Here's how the part is built. I have some questions about the finished solid (model axes, mm). A direction names the side the tool comes from. Round coordinates to 2 decimals unless told otherwise and drop trailing zeros. Order: outer loops, then holes, each group sorted by start corner. A loop starts at its lowest first (then second) coordinate and runs counter-clockwise, first axis right, second up.
```python
from build123d import *

# Parameters (mm, degrees)
SKETCH1_R           = 14
SKETCH1_R_2         = 5
BOSS_EXTRUDE1_DEPTH = 38
SKETCH2_R           = 6.35
SKETCH2_R_2         = 3.25
BOSS_EXTRUDE2_DEPTH = 12
SKETCH3_R           = 2.5
CUT_EXTRUDE6_DEPTH  = 10


with BuildPart() as part:
    # Sketch1 → Boss-Extrude1 (new body)
    with BuildSketch(Plane(origin=(0, 0, 0), x_dir=(1, 0, 0), z_dir=(0, 1, 0))):
        with BuildLine():
            Line((40, 57), (-40, 57))
            ThreePointArc((-40, 57), (-58.987886037, 46.111263827), (-59.17994648, 24.223653075))
            Line((-59.17994648, 24.223653075), (-47.255332989, 3))
            Line((-47.255332989, 3), (-32.311027529, 3))
            ThreePointArc((-32.311027529, 3), (32.415238263, -1.501608583), (-32.45, 0))
            Line((-32.45, 0), (-47.255332989, 0))
            Line((-47.255332989, 0), (-47.255332989, -10))
            Line((-47.255332989, -10), (-41.255332989, -10))
            ThreePointArc((-41.255332989, -10), (-4.643586709, -42.195255687), (38.093342034, -18.732319468))
            Line((38.093342034, -18.732319468), (59.742132503, 25.291848568))
            ThreePointArc((59.742132503, 25.291848568), (58.675911377, 46.627997861), (40, 57))
        make_face()
        with Locations((-40, 35)):
            Circle(SKETCH1_R, mode=Mode.SUBTRACT)
        with Locations((0, 44)):
            Circle(SKETCH1_R_2, mode=Mode.SUBTRACT)
        with Locations((40, 35)):
            Circle(SKETCH1_R, mode=Mode.SUBTRACT)
    extrude(amount=BOSS_EXTRUDE1_DEPTH)


with BuildPart() as body_2:
    # Sketch2 → Boss-Extrude2 (new body)
    with BuildSketch(Plane(origin=(0, 38, 0), x_dir=(1, 0, 0), z_dir=(0, 1, 0))):
        with BuildLine():
            Line((-40, 27), (40, 27))
            ThreePointArc((40, 27), (45.282843577, 28.992374534), (47.934336402, 33.977109066))
            Line((47.934336402, 33.977109066), (50, 50))
            Line((50, 50), (50, 58))
            Line((50, 58), (-50, 58))
            Line((-50, 58), (-50, 50))
            Line((-50, 50), (-47.934336402, 33.977109066))
            ThreePointArc((-47.934336402, 33.977109066), (-45.282843577, 28.992374534), (-40, 27))
        make_face()
        with Locations((0, 44)):
            Circle(SKETCH2_R, mode=Mode.SUBTRACT)
        with Locations((-40, 35)):
            Circle(SKETCH2_R_2, mode=Mode.SUBTRACT)
        with Locations((40, 35)):
            Circle(SKETCH2_R_2, mode=Mode.SUBTRACT)
    extrude(amount=BOSS_EXTRUDE2_DEPTH)

    # Sketch3 → Cut-Extrude6 (cut)
    with BuildSketch(Plane(origin=(0, 0, -58), x_dir=(-1, 0, 0), z_dir=(0, 0, -1))):
        with Locations((0, 44)):
            Circle(SKETCH3_R)
        with Locations((40, 44)):
            Circle(SKETCH3_R)
        with Locations((-40, 44)):
            Circle(SKETCH3_R)
    extrude(amount=-CUT_EXTRUDE6_DEPTH, mode=Mode.SUBTRACT)


solid = body_2.part
```
1) We'd pull the mould along Y, two halves only. Please class faces 1 (the cylindrical face through (-38.5, 43.916, -32.117)), 2 (the flat face through (-1, 50, -36)), 3 (the flat face through (-40, 44, -48)): +Y half, -Y half, draft (parallel to the pull), parting line (faces both ways), or undercut.
2) I need wall thicknesses on line 1 (Z direction, x = 0, y = 41.25); line 2 (Y direction, x = -40, z = -54); line 3 (X direction, y = 49.75, z = -36.5). Which ranges of each line are inside material? Lowest first, please.
3) If we section it at D-D (y = 44): Write out the boundary of the cut face in (x, z).
4) I'm going to push flat-ended pins straight in: pin 1 (16.5 mm diameter, centred on x = 0, z = -44, fed in from -Y); pin 2 (1 mm diameter, centred on y = 44, z = -46, fed in from -X); pin 3 (4 mm diameter, centred on y = 43, z = -38.5, fed in from +X); pin 4 (2.5 mm diameter, centred on x = 40.5, y = 44.5, fed in from -Z). Where does each tip first touch, or does it pass through?
5) If we section it at B-B (x = 0): Write out the boundary of the cut face in (y, z), plus the area to 3 significant figures.
6) If we section it at A-A (z = -53): Write out the boundary of the cut face in (x, y), plus the area to 3 significant figures.
7) For faces 4 (the flat face through (-48.98, 43.92, -42.1)), 5 (the cylindrical face through (37.69, 43.04, -53.07)), which set-ups out of +Z, -Z, +X, -X, +Y, -Y let a thin tool reach every point of the face, with its end or its side?
8) If we section it at C-C (y = 48.25): Write out the boundary of the cut face in (x, z), plus the area to 3 significant figures.
Solutions:
1. face 1: draft
1. face 2: +Y half
1. face 3: undercut
2. line 1: z = -58 to -50.35, -37.65 to -27
2. line 2: y = 38 to 41.5, 46.5 to 50
2. line 3: x = -48.26 to -42.88, -37.12 to 37.12, 42.88 to 48.26
3. outline: (-50, -58) - (-42.5, -58) - (-42.5, -48) - (-37.5, -48) - (-37.5, -58) - (-2.5, -58) - (-2.5, -49.84) arc R6.35 cw (long way) to (2.5, -49.84) - (2.5, -58) - (37.5, -58) - (37.5, -48) - (42.5, -48) - (42.5, -58) - (50, -58) - (50, -50) - (47.93, -33.98) arc R8 ccw to (40, -27) - (-40, -27) arc R8 ccw to (-47.93, -33.98) - (-50, -50) - close; hole circle Ø6.5 at (-40, -35); hole circle Ø6.5 at (40, -35)
4. pin 1: stops at y = 38
4. pin 2: stops at x = -49.55
4. pin 3: stops at x = 48.78
4. pin 4: stops at z = -48
5. outline: (38, -58) - (41.5, -58) - (41.5, -50.35) - (38, -50.35) - close; (38, -37.65) - (50, -37.65) - (50, -27) - (38, -27) - close; (46.5, -58) - (50, -58) - (50, -50.35) - (46.5, -50.35) - close
5. area: 181 mm2
6. outline: (-50, 38) - (50, 38) - (50, 50) - (-50, 50) - close; hole circle Ø5 at (-40, 44); hole circle Ø5 at (0, 44); hole circle Ø5 at (40, 44)
6. area: 1,140 mm2
7. face 4: +Z, -X, +Y, -Y
7. face 5: -Z
8. outline: (-50, -58) - (50, -58) - (50, -50) - (47.93, -33.98) arc R8 ccw to (40, -27) - (-40, -27) arc R8 ccw to (-47.93, -33.98) - (-50, -50) - close; hole circle Ø6.5 at (-40, -35); hole circle Ø12.7 at (0, -44); hole circle Ø6.5 at (40, -35)
8. area: 2,820 mm2
